```python
from build123d import *

# Parameters (mm, degrees)
SKETCH1_W                = 33.02
SKETCH1_H                = 25.4
BOSS_EXTRUDE1_DEPTH      = 4
SKETCH2_W                = 33.02
SKETCH2_H                = 19.05
BOSS_EXTRUDE2_DEPTH      = 13.320199928
BOSS_EXTRUDE3_DEPTH      = 33.02
F_0_257_DIAMETER_HOLE1_D = 6.5278
CUT_EXTRUDE1_DEPTH       = 7.62
M2_CLEARANCE_HOLE1_D     = 2.6
CHAMFER1_SIZE            = 1


with BuildPart() as part:
    # Sketch1 → Boss-Extrude1 (new body)
    with BuildSketch(Plane(origin=(0, 0, 0), x_dir=(0, 0, -1), z_dir=(1, 0, 0))):
        with Locations((16.51, -12.7)):
            Rectangle(SKETCH1_W, SKETCH1_H)
    extrude(amount=BOSS_EXTRUDE1_DEPTH)



with BuildPart() as body_2:
    # Sketch2 → Boss-Extrude2 (new body)
    with BuildSketch(Plane(origin=(4, 0, 0), x_dir=(0, 0, -1), z_dir=(1, 0, 0))):
        with Locations((16.51, 9.525)):
            Rectangle(SKETCH2_W, SKETCH2_H)
    extrude(amount=BOSS_EXTRUDE2_DEPTH)


with BuildPart() as part_1:
    add(part.part)

    add(body_2.part)  # Boss-Extrude3 merges body 2
    # Sketch3 → Boss-Extrude3 (add)
    with BuildSketch(Plane.XY):
        Polygon((4, 19.05), (0, 0), (4, 0), align=None)
    extrude(amount=-BOSS_EXTRUDE3_DEPTH)

    # F (0.257) Diameter Hole1 (through all)
    with Locations(Plane(origin=(17.320199928, 0, 0), x_dir=(0, 0, -1), z_dir=(1, 0, 0))):
        with Locations((7.62, 9.525), (25.4, 9.525)):
            Hole(F_0_257_DIAMETER_HOLE1_D / 2)

    # Sketch11 → Cut-Extrude1 (cut)
    with BuildSketch(Plane.ZY):
        with BuildLine():
            Line((-25.4, 15.113), (-7.62, 15.113))
            ThreePointArc((-7.62, 15.113), (-2.032, 9.525), (-7.62, 3.937))
            Line((-7.62, 3.937), (-25.4, 3.937))
            ThreePointArc((-25.4, 3.937), (-30.988, 9.525), (-25.4, 15.113))
        make_face()
    extrude(amount=-CUT_EXTRUDE1_DEPTH, mode=Mode.SUBTRACT)

    # M2 Clearance Hole1 (through all)
    with Locations(Plane.ZY):
        with Locations((-16.51, -6.9), (-16.51, -18.5)):
            Hole(M2_CLEARANCE_HOLE1_D / 2)

    # Chamfer1
    chamfer1_edges = [part_1.edges().sort_by_distance(p)[0] for p in [
        (4, 0, -16.51),
    ]]
    chamfer(chamfer1_edges, length=CHAMFER1_SIZE)


solid = part_1.part
```
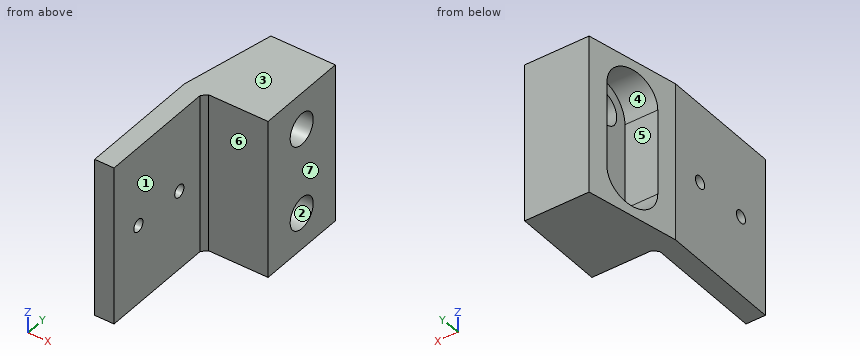
CAD build for the part. Positions are in the model's coordinates, mm. Face numbers are marked on the shaded views. A direction names the side the tool comes from. Coordinates: 2 decimals unless noted, no trailing zeros. Write each loop counter-clockwise with the first axis right and the second up, starting at its lowest first coordinate (ties: lowest second). Pieces come first, ordered by that corner, then holes.
(1) Two-plate mould, pull along Z, no slides. Class the marked faces 1, 2, 3 and 4: +Z half, -Z half, draft (parallel to the pull), parting line (faces both ways), or undercut.
(2) 3-axis set-ups, long thin cutter, end or side, ignore diameter. For the marked faces 5, 6 and 7: which of +Z, -Z, +X, -X, +Y, -Y reach the whole face in a straight line?
(3) Flat gauge pins, fed straight in: pin 1 (7.5 mm diameter, centred on y = -17.5, z = -13.5, fed in from +X); pin 2 (3.5 mm diameter, centred on x = 14, z = -17, fed in from -Y); pin 3 (8 mm diameter, centred on y = 7, z = -12.5, fed in from -X). Where does each tip first touch, or does it go through?
(4) Cut at C-C, the plane x = 6.5. List the corners of the cut face in (y, z) (3 decimals).
(5) Cut at D-D, the plane z = -10. List the corners of the cut face in (x, y).
(6) Cut at B-B, the plane z = -16.51. List the corners of the cut face in (x, y), and give its area (3 significant figures).
(7) Drill centre lines: probe 1 along Y at (x, z) = (2.1, -16.51); probe 2 along Y at (x, z) = (13.75, -25.4); probe 3 along X at (y, z) = (-8.5, -17). Where is each one in solid material? Low to high.
(8) Cut at A-A, the plane y = -18.5. List the corners of the cut face in (x, z).
Geometry says:
1. face 1: draft
1. face 2: undercut
1. face 3: +Z half
1. face 4: undercut
2. face 5: -X
2. face 6: +Z, -Z, +X, -Y
2. face 7: +Z, -Z, +X, +Y, -Y
3. pin 1: stops at x = 4
3. pin 2: stops at y = 0
3. pin 3: stops at x = 0.63
4. outline: (0, -33.02) - (19.05, -33.02) - (19.05, 0) - (0, 0) - close; hole (3.937, -25.4) arc R5.588 ccw to (15.113, -25.4) - (15.113, -7.62) arc R5.588 ccw to (3.937, -7.62) - close
5. outline: (0, -25.4) - (4, -25.4) - (4, -1) - (5, 0) - (17.32, 0) - (17.32, 7.29) - (7.62, 7.29) - (7.62, 3.94) - (0.83, 3.94) - (0, 0) - close; (3.17, 15.11) - (7.62, 15.11) - (7.62, 11.76) - (17.32, 11.76) - (17.32, 19.05) - (4, 19.05) - close
6. outline: (0, -25.4) - (4, -25.4) - (4, -19.8) - (0, -19.8) - close; (0, -17.2) - (4, -17.2) - (4, -8.2) - (0, -8.2) - close; (0, -5.6) - (4, -5.6) - (4, -1) - (5, 0) - (17.32, 0) - (17.32, 19.05) - (4, 19.05) - (3.17, 15.11) - (7.62, 15.11) - (7.62, 3.94) - (0.83, 3.94) - (0, 0) - close
6. area: 310 mm2
7. probe 1: y = -25.4 to -19.8, -17.2 to -8.2, -5.6 to 3.94
7. probe 2: y = 0 to 6.26, 12.79 to 19.05
7. probe 3: x = 0 to 4
8. outline: (0, -33.02) - (4, -33.02) - (4, -17.81) - (0, -17.81) - close; (0, -15.21) - (4, -15.21) - (4, 0) - (0, 0) - close
